Autodesk Inventor part; units mm, degrees
ref_plane "Work Plane1" through (0, 0, 10) normal (0, 0, 1) x (1, 0, 0)
ref_plane "Work Plane3" through (3.9701, 45.8299, 26) normal (1, 0, 0) x (0, -1, 0)
ref_plane "Work Plane4" through (-34.8055, 8.3289, 16.6138) normal (0.7071068, -0.7071068, 0) x (0.7071068, 0.7071068, 0)
ref_plane "Work Plane1" through (0, 0, 10) normal (0, 0, 1) x (1, 0, 0)
sketch "Sketch1" plane through (0, 0, 10) normal (0, 0, 1) x (1, 0, 0)
  line L0 (-4.0299, -0.3538) -> (-2.2322, 1.4439) construction
  arc A0 (-1.4439, 2.2322) -> (-2.2322, 1.4439) centre (-0.9299, 0.9299) ccw construction
  line L1 (-1.4439, 2.2322) -> (0.3538, 4.0299) construction
  line L2 (-37.8299, 42.8299) -> (-37.8299, 37.8299) construction
  line L3 (-37.8299, 37.8299) -> (-42.9208, 37.8299) construction
  line L4 (-37.8299, 42.2137) -> (-37.8299, 45.8299) construction
  line L5 (-37.8299, 45.8299) -> (-4.0299, 45.8299) construction
  line L6 (-4.0299, 45.8299) -> (-4.0299, 42.2137) construction
  line L7 (-4.0299, 4.0299) -> (0.3538, 4.0299)
  circle A1 centre (-20.9299, 20.9299) radius 17.5
  line L8 (-20.9299, 58.9723) -> (17.1124, 20.9299) construction
  line L9 (17.1124, 20.9299) -> (-20.9299, -17.1124) construction
  line L10 (-20.9299, -17.1124) -> (-58.9723, 20.9299) construction
  line L11 (-58.9723, 20.9299) -> (-20.9299, 58.9723) construction
  line L12 (-20.9299, 58.9723) -> (-20.9299, -17.1124) construction
  line L13 (17.1124, 20.9299) -> (-58.9723, 20.9299) construction
  line L14 (-20.9299, 58.9723) -> (32.8701, 58.9723) construction
  line L15 (-43.4299, 43.4299) -> (1.5701, 43.4299) construction
  line L16 (1.5701, 43.4299) -> (1.5701, -1.5701) construction
  line L17 (1.5701, -1.5701) -> (-43.4299, -1.5701) construction
  line L18 (-43.4299, -1.5701) -> (-43.4299, 43.4299) construction
  line L19 (-43.4299, 43.4299) -> (1.5701, -1.5701) construction
  line L20 (1.5701, 43.4299) -> (-43.4299, -1.5701) construction
  line L21 (-43.4299, 5.3876) -> (-43.4299, 36.4723)
  line L22 (-43.4299, 36.4723) -> (-36.4723, 43.4299)
  line L23 (-36.4723, 43.4299) -> (-5.3876, 43.4299)
  line L24 (-5.3876, 43.4299) -> (1.5701, 36.4723)
  line L25 (1.5701, 36.4723) -> (1.5701, 5.3876)
  line L26 (1.5701, 5.3876) -> (-5.3876, -1.5701)
  line L27 (-5.3876, -1.5701) -> (-36.4723, -1.5701)
  line L28 (-36.4723, -1.5701) -> (-43.4299, 5.3876)
  line L29 (-4.0299, 42.2137) -> (-37.8299, 42.2137)
  line L30 (-4.0299, -0.3538) -> (-4.0299, 4.0299)
  circle A2 centre (-20.9299, 20.9299) radius 1.4
  line L31 (-10.9299, 10.9299) -> (-30.9299, 10.9299) construction
  line L32 (-30.9299, 10.9299) -> (-30.9299, 30.9299) construction
  line L33 (-30.9299, 30.9299) -> (-10.9299, 30.9299) construction
  line L34 (-10.9299, 30.9299) -> (-10.9299, 10.9299) construction
  line L35 (-10.9299, 10.9299) -> (-30.9299, 30.9299) construction
  line L36 (-30.9299, 10.9299) -> (-10.9299, 30.9299) construction
  circle A3 centre (-30.9299, 30.9299) radius 1.4
  circle A4 centre (-30.9299, 10.9299) radius 1.4
  circle A5 centre (-10.9299, 10.9299) radius 1.4
  line L37 (-45.8299, 37.8299) -> (-42.0723, 37.8299) construction
  line L38 (-42.1723, 37.7299) -> (-45.8299, 37.7299)
  line L39 (-45.8299, 37.7299) -> (-45.8299, 4.1299)
  line L40 (-45.8299, 4.1299) -> (-42.1723, 4.1299)
  line L41 (-42.1723, 4.1299) -> (-42.1723, 37.7299)
  line L42 (-45.8299, 4.0299) -> (-42.0723, 4.0299) construction
  line L43 (-45.8299, 37.8299) -> (-42.0723, 37.8299)
  line L44 (-37.7299, 45.8299) -> (-4.1299, 45.8299)
  line L45 (-4.1299, 45.8299) -> (-4.1299, 42.1723)
  line L46 (-4.1299, 42.1723) -> (-37.7299, 42.1723)
  line L47 (-37.7299, 42.1723) -> (-37.7299, 45.8299)
  line L48 (0.4701, 37.8299) -> (0.4701, 4.0299) construction
  line L49 (0.4701, 4.0299) -> (3.9701, 4.0299) construction
  line L50 (3.9701, 37.8299) -> (3.9701, 4.0299) construction
  line L51 (0.4701, 37.8299) -> (3.9701, 37.8299) construction
  line L52 (-45.8299, -3.9701) -> (-4.0299, -3.9701) construction
  line L53 (0.3124, 37.7299) -> (3.9701, 37.7299)
  line L54 (3.9701, 37.7299) -> (3.9701, 4.1299)
  line L55 (3.9701, 4.1299) -> (0.3124, 4.1299)
  line L56 (0.3124, 4.1299) -> (0.3124, 37.7299)
  line L57 (-4.1713, -0.3538) -> (-37.7299, -0.3538)
  line L58 (-37.7299, -0.3538) -> (-37.7299, -3.9701)
  line L59 (-37.7299, -3.9701) -> (-4.1713, -3.9701)
  line L60 (-4.1713, -3.9701) -> (-4.1713, -0.3538)
  point P0 (-37.8299, 4.0299)
  dimension "d18" = 53.8
  dimension "d19" = 45
  dimension "d20" = 53.8
  dimension "d21" = 45
  dimension "d22" = 45
  dimension "d30" = 20
  dimension "d31" = 20
  dimension "d32" = 2.8
  dimension "d33" = 2.8
  dimension "d34" = 2.8
  dimension "d35" = 2.8
  dimension "d36" = 0.1
  dimension "d37" = 0.1
  dimension "d38" = 0.1
  dimension "d39" = 0.1
extrude "Extrusion1" add sketch "Sketch1" along normal blind 5 contours L30 L26 L57 L28 L41 L22 L46 L24 L56 L7 | L7 L26 L30 | L56 L24 L25 L26 | L26 L25 L24 L53 L54 L55 | L60 L59 L58 L57 L28 L27 L26 | L26 L27 L28 L57 | L46 L22 L29 L24 | L24 L29 L45 | L40 L39 L38 L22 L21 L28 | L28 L21 L22 L41 | L29 L22 L23 L24 | L24 L23 L22 L29 L47 L44 L45 | L47 L29 L22 | A1 | A2 | A3 | A4 | A5
sketch "Sketch4" plane through (0, 0, 15) normal (0, 0, 1) x (1, 0, 0)
  line L0 (-37.7299, 42.1723) -> (-42.1723, 37.7299)
  line L1 (-42.1723, 37.7299) -> (-45.8299, 37.7299)
  line L2 (-45.8299, 37.7299) -> (-45.8299, 4.1299)
  line L3 (-45.8299, 4.1299) -> (-42.1723, 4.1299)
  line L4 (-42.1723, 4.1299) -> (-37.6885, -0.3538)
  line L5 (-37.6885, -0.3538) -> (-37.7299, -0.3538)
  line L6 (-37.7299, -0.3538) -> (-37.7299, -3.9701)
  line L7 (-37.7299, -3.9701) -> (-4.1713, -3.9701)
  line L8 (-4.1713, -3.9701) -> (-4.1713, -0.3538)
  line L9 (-4.1713, -0.3538) -> (0.3124, 4.1299)
  line L10 (0.3124, 4.1299) -> (3.9701, 4.1299)
  line L11 (3.9701, 4.1299) -> (3.9701, 37.7299)
  line L12 (3.9701, 37.7299) -> (0.3124, 37.7299)
  line L13 (0.3124, 37.7299) -> (-4.1299, 42.1723)
  line L14 (-4.1299, 42.1723) -> (-4.1299, 45.8299)
  line L15 (-4.1299, 45.8299) -> (-37.7299, 45.8299)
  line L16 (-37.7299, 45.8299) -> (-37.7299, 42.1723)
  line L17 (-45.8299, 37.7299) -> (-45.8299, 4.1299)
  line L18 (-45.8299, 7.911) -> (-7.911, 45.8299)
  line L19 (-45.8299, 7.911) -> (7.7955, 7.911) construction
  line L20 (-7.911, 45.8299) -> (-14.9821, 45.8299)
  line L21 (-4.1299, 45.8299) -> (-37.7299, 45.8299)
  line L22 (-14.9821, 45.8299) -> (-45.8299, 14.9821)
  line L23 (-45.8299, 7.911) -> (-45.8299, 14.9821)
  circle A0 centre (-40.9299, 0.9299) radius 1.1933
  circle A1 centre (-0.9299, 40.9299) radius 1.4
  line L24 (-40.9299, 0.9299) -> (-0.9299, 40.9299)
  line L25 (0.3124, 37.7299) -> (-4.1299, 42.1723)
  point P0 (0, 0)
  dimension "d40" = 45
  dimension "d41" = 5
extrude "Extrusion4" add sketch "Sketch4" along normal blind 27.5 contours L15 L18 L2 L22
sketch "Sketch5" plane through (-45.8299, 14.9821, 15) normal (-0.7071068, 0.7071068, 0) x (-0.7071068, -0.7071068, 0)
  line L0 (0, 0) -> (-43.6254, 0)
  line L1 (0, 0) -> (0, 27.5)
  line L2 (-43.6254, 27.5) -> (0, 27.5)
  line L3 (-43.6254, 0) -> (-43.6254, 27.5)
  circle A0 centre (-21.8127, 5.6873) radius 21.8127
  line L4 (-6.8127, 24) -> (-36.8127, 24) construction
  line L5 (-36.8127, 24) -> (-36.8127, 4) construction
  line L6 (-36.8127, 4) -> (-6.8127, 4) construction
  line L7 (-6.8127, 4) -> (-6.8127, 24) construction
  line L8 (-6.8127, 24) -> (-36.8127, 4) construction
  line L9 (-36.8127, 24) -> (-6.8127, 4) construction
  point P0 (-21.8127, -15)
  point P1 (-21.8127, 14)
  dimension "d44" = 30
  dimension "d45" = 20
hole "Hole1" at (-19.7994, 41.0126, 39) at (-19.7994, 41.0126, 19) at (-41.0126, 19.7994, 39) at (-30.406, 30.406, 29) direction (0.7071068, -0.7071068, 0) diameter 2.8 depth 12
sketch "Sketch6" plane through (-37.7299, -3.9701, 10) normal (0, -1, 0) x (1, 0, 0)
  circle A0 centre (-3.2, 36.9) radius 1.45
  circle A1 centre (36.8, 36.9) radius 1.45
  line L0 (-6.1, 0) -> (-6.1, 39.8)
  line L1 (-0.1, 0) -> (-6.1, 0)
  line L2 (-0.1, 33.8) -> (-0.1, 0)
  line L3 (33.7, 33.8) -> (-0.1, 33.8)
  line L4 (33.7, 33.8) -> (33.7, 0)
  line L5 (39.7, 0) -> (33.7, 0)
  line L6 (39.7, 39.8) -> (39.7, 0)
  line L7 (-6.1, 39.8) -> (39.7, 39.8)
  circle A2 centre (16.8, 16.9) radius 16.9
  circle A3 centre (16.8, 16.9) radius 14.9
  line L8 (-0.1, 16.9) -> (-0.1, 0)
  line L9 (0, 0) -> (33.5586, 0)
  line L10 (0.0414, 0) -> (-4.4423, 0)
  line L11 (33.5586, 0) -> (0.0414, 0)
  line L12 (33.7, 16.9) -> (33.5586, 0)
  point P0 (37.7299, -10)
  dimension "d53" = 2
extrude "Extrusion5" cut sketch "Sketch6" against normal up to surface contours A3 surface through (-45.8299, 7.911, 15) normal (0.7071068, -0.7071068, 0)
ref_plane "Work Plane3" through (3.9701, 45.8299, 26) normal (1, 0, 0) x (0, -1, 0)
sketch "Sketch7" plane through (3.9701, 45.8299, 26) normal (1, 0, 0) x (0, -1, 0)
  line L0 (41.8, -17.8) -> (41.8, 16)
  line L1 (8, -17.8) -> (41.8, -17.8)
  line L2 (8, -17.8) -> (8, 16)
  circle A0 centre (24.9, -0.9) radius 16.9
  circle A1 centre (24.9, -0.9) radius 14.9
  point P0 (45.8299, 26)
  dimension "d56" = 2
ref_plane "Work Plane4" through (-34.8055, 8.3289, 16.6138) normal (0.7071068, -0.7071068, 0) x (0.7071068, 0.7071068, 0)
extrude "Extrusion6" cut sketch "Sketch7" against normal up to surface contours A1 surface through (-45.8299, 7.911, 15) normal (0.7071068, -0.7071068, 0)
sketch "Skizze8" plane through (0, 0, 10) normal (0, 0, -1) x (-1, 0, 0)
  line L0 (42.1723, 37.7299) -> (37.7299, 42.1723)
  line L1 (37.7299, 45.8299) -> (37.7299, 42.1723)
  line L2 (4.1299, 45.8299) -> (37.7299, 45.8299) construction
  line L3 (4.1299, 42.1723) -> (4.1299, 45.8299)
  line L4 (4.1299, 42.1723) -> (-0.3124, 37.7299)
  line L5 (-3.9701, 37.7299) -> (-0.3124, 37.7299)
  line L6 (-3.9701, 4.1299) -> (-3.9701, 37.7299) construction
  line L7 (-0.3124, 4.1299) -> (-3.9701, 4.1299)
  line L8 (-0.3124, 4.1299) -> (4.1713, -0.3538)
  line L9 (4.1713, -3.9701) -> (4.1713, -0.3538)
  line L10 (37.7299, -3.9701) -> (4.1713, -3.9701) construction
  line L11 (37.7299, -0.3538) -> (37.7299, -3.9701)
  line L12 (37.6885, -0.3538) -> (37.7299, -0.3538)
  line L13 (37.6885, -0.3538) -> (42.1723, 4.1299)
  line L14 (45.8299, 4.1299) -> (42.1723, 4.1299)
  line L15 (45.8299, 37.7299) -> (45.8299, 4.1299) construction
  line L16 (42.1723, 37.7299) -> (45.8299, 37.7299)
  line L17 (45.9299, 4.0299) -> (42.2137, 4.0299)
  line L18 (42.2137, 4.0299) -> (37.8299, -0.3538)
  line L19 (37.8299, -0.3538) -> (37.8299, -4.0701)
  line L20 (37.8299, -4.0701) -> (4.0713, -4.0701) construction
  line L21 (4.0713, -4.0701) -> (4.0713, -0.3953)
  line L22 (4.0713, -0.3953) -> (-0.3538, 4.0299)
  line L23 (-0.3538, 4.0299) -> (-4.0701, 4.0299)
  line L24 (-4.0701, 4.0299) -> (-4.0701, 37.8299) construction
  line L25 (-4.0701, 37.8299) -> (-0.3538, 37.8299)
  line L26 (-0.3538, 37.8299) -> (4.0299, 42.2137)
  line L27 (4.0299, 42.2137) -> (4.0299, 45.9299)
  line L28 (4.0299, 45.9299) -> (37.8299, 45.9299) construction
  line L29 (37.8299, 45.9299) -> (37.8299, 42.2137)
  line L30 (37.8299, 42.2137) -> (42.2137, 37.8299)
  line L31 (42.2137, 37.8299) -> (45.9299, 37.8299)
  line L32 (45.9299, 37.8299) -> (45.9299, 4.0299) construction
  line L33 (37.7299, 45.8299) -> (37.7299, 42.1723)
  line L34 (37.7299, 45.8299) -> (37.8299, 45.8299)
  line L35 (42.1723, 37.7299) -> (45.8299, 37.7299)
  line L36 (45.8299, 37.7299) -> (45.8299, 37.8299)
  line L37 (45.8299, 4.1299) -> (45.8299, 4.0299)
  line L38 (37.7299, -3.9701) -> (4.1713, -3.9701)
  line L39 (37.7299, -3.9701) -> (37.8299, -3.9701)
  line L40 (4.1713, -3.9701) -> (4.0713, -3.9701)
  line L41 (-3.9701, 4.1299) -> (-3.9701, 4.0299)
  line L42 (-3.9701, 37.7299) -> (-0.3124, 37.7299)
  line L43 (-3.9701, 37.7299) -> (-3.9701, 37.8299)
  line L44 (4.1299, 42.1723) -> (4.1299, 45.8299)
  line L45 (4.1299, 45.8299) -> (4.0299, 45.8299)
  point P0 (0, 0)
  dimension "d59" = 0.1
extrude "IM_offset" add sketch "Skizze8" against normal up to surface (5 mm away)
properties part number "20_Cube_Insert_Kinematic_Mirrormount_45_base_v3_aaa"
Build history of the part. All positions in model axes, mm. A direction names the side the tool comes from. Coordinates: 2 decimals unless noted, no trailing zeros. Write each loop counter-clockwise with the first axis right and the second up, starting at its lowest first coordinate (ties: lowest second). Pieces come first, ordered by that corner, then holes.
1. Drop flat-ended pins along their axis: pin 1 (1.1 mm diameter, centred on x = -45, z = 13, fed in from +Y); pin 2 (1 mm diameter, centred on x = -7, z = 37.5, fed in from +Y); pin 3 (1.8 mm diameter, centred on y = -2, z = 11.5, fed in from +X); pin 4 (3 mm diameter, centred on x = -44.5, z = 12, fed in from -Y). Give the stop position or say it passes through.
Answer block:
pin 1: stops at y = 37.83
pin 2: passes through
pin 3: stops at x = -4.07
pin 4: stops at y = 4.03
2. Band-saw the part on D-D, the plane x = -32.5. Give the cut face in (y, z).
Answer block:
outline: (-3.97, 10) - (45.83, 10) - (45.83, 15) - (28.31, 15) - (28.31, 42.5) - (21.24, 42.5) - (21.24, 12) arc R14.9 cw to (11.96, 15) - (-3.97, 15) - close
3. Drill centre lines: probe 1 along Z at (x, y) = (-32, 1); probe 2 along Z at (x, y) = (-19, 21); probe 3 along X at (y, z) = (-2, 13.5). Where is each one in solid material? Low to high.
Answer block:
probe 1: z = 10 to 15
probe 2: z = 10 to 12
probe 3: x = -37.83 to -27.45, -14.41 to -4.07
4. Band-saw the part on A-A, the plane x = -6. Give the cut face in (y, z).
Answer block:
outline: (-3.97, 10) - (45.83, 10) - (45.83, 15) - (29.9, 15) arc R14.9 cw to (11.96, 15) - (-3.97, 15) - close
5. Pull direction Y, two halves, no side cores. Call faces 4 (the cylindrical face through (-17.04, 40.19, 18.7)), 5 (the flat face through (-6, 36, 15)), 6 (the flat face through (-21, -3.97, 11)): released by +Y, released by -Y, zero draft, split by the parting line, or undercut.
Answer block:
face 4: undercut
face 5: zero draft
face 6: released by -Y
6. Band-saw the part on C-C, the plane y = 40. Give the number of separate pieces and of enclosed holes in the cut face, and give its area (3 significant figures).
Answer block:
separate pieces: 1
enclosed holes: 2
area: 367 mm2
7. Band-saw the part on B-B, the plane z = 26.5. Give the cut face in (x, y), and give its area (3 significant figures).
Answer block:
outline: (-45.83, 7.91) - (-7.91, 45.83) - (-14.98, 45.83) - (-45.83, 14.98) - close
area: 243 mm2
8. 3-axis set-ups, long thin cutter, end or side, ignore diameter. For faces 1 (the flat face through (-37.83, -2, 12)), 2 (the flat face through (-30.19, 30.62, 25.5)), 3 (the cylindrical face through (-17.566, 31.208, 12.385)): which of +Z, -Z, +X, -X, +Y, -Y reach the whole face in a straight line?
Answer block:
face 1: +Z, -Z, -X, -Y
face 2: +Z, -X, +Y
face 3: +Z, -Y
